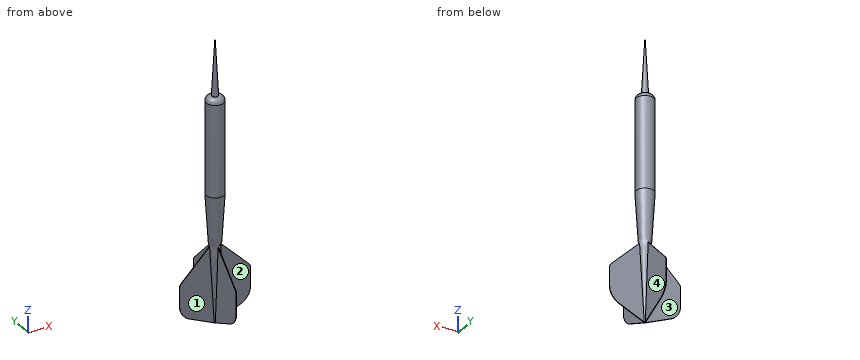
```python
from build123d import *

# Parameters (mm, degrees)
FLIGHT_DEPTH  = 0.125
FLIGHTS_COUNT = 4


with BuildPart() as part:
    # Sketch1 → Dart (revolve)
    with BuildSketch(Plane(origin=(0, 0, 0), x_dir=(0, 0, -1), z_dir=(1, 0, 0))):
        with BuildLine():
            Line((0, 0), (-32, 0))
            Line((-32, 0), (0, 1.75))
            ThreePointArc((0, 1.75), (0.787661698, 3.896312185), (2.887760572, 4.8))
            Line((2.887760572, 4.8), (52.94, 4.8))
            Line((52.94, 4.8), (122.94, 0.5))
            Line((122.94, 0.5), (122.94, 0))
            Line((122.94, 0), (0, 0))
        make_face()
    revolve(axis=Axis((0, 0, -122.94), (0, 0, 1)))

    # Sketch3 → Flight (add, symmetric)
    with BuildSketch(Plane(origin=(0, 0, 0), x_dir=(0, 0, -1), z_dir=(1, 0, 0))):
        with BuildLine():
            Line((77.94, 0), (96.561320344, 18.621320344))
            ThreePointArc((96.561320344, 18.621320344), (97.53459039, 19.271638598), (98.682640687, 19.5))
            Line((98.682640687, 19.5), (108.63598664, 19.5))
            ThreePointArc((108.63598664, 19.5), (113.537737955, 18.048035112), (116.857895759, 14.160629788))
            Line((116.857895759, 14.160629788), (122.94, 0.5))
            Line((122.94, 0.5), (122.94, 0))
            Line((122.94, 0), (77.94, 0))
        make_face()
    flight = extrude(amount=FLIGHT_DEPTH, both=True)

    # Flights: Flight ×4 about axis
    flights_axis = Axis((0, 0, 0), (0, 0, 1))
    for i in range(1, FLIGHTS_COUNT):
        add(flight.rotate(flights_axis, i * 360 / FLIGHTS_COUNT))


solid = part.part
```
Work out the finished part from the listing and answer in its coordinate system (mm). Face numbers are marked on the shaded views. A direction names the side the tool comes from. Give positions to 0.01 mm unless a question says otherwise; leave off trailing zeros. Write each loop counter-clockwise with the first axis right and the second up, starting at its lowest first coordinate (ties: lowest second). Pieces come first, ordered by that corner, then holes. Notation, with made-up numbers: (29.5, 51.5) - (86.5, 51.5) arc R27 cw to (86.5, 69.5) - close; hole circle Ø3 at (-27, -22). An arc over 180 degrees is marked (long way). Use one line per item in the form item = value.
1. Consider L1, parallel to Y at x = -8, z = -87 (3 decimals); L2, parallel to X at y = 0.5, z = -44. Determine where each line is inside the solid, lowest interval first.
Filled in:
L1 = -0.125 to 0.125
L2 = -4.77 to 4.77
2. A cutting plane is placed at A-A (y = 9.5). Write down the section's boundary in (x, z) (3 decimals).
Filled in:
outline = (-0.125, -118.933) - (0.125, -118.933) - (0.125, -87.44) - (-0.125, -87.44) - close
3. A cutting plane is placed at C-C (z = -38). Write down the section's boundary in (x, y).
Filled in:
outline = circle Ø9.6 at (0, 0)
4. For the marked faces 1, 2, 3 and 4, determine the directions among +Z, -Z, +X, -X, +Y, -Y from which every point of the face is accessible in a straight line to the end or side of a thin tool.
Filled in:
face_1 = -Z, -X, -Y
face_2 = -Z, +X, -Y
face_3 = -Z, -X, +Y
face_4 = -Z, +X, +Y
5. A cutting plane is placed at B-B (z = -75.5). Write down the section's boundary in (x, y), and give its area (3 significant figures).
Filled in:
outline = circle Ø6.83 at (0, 0)
area = 36.6 mm^2
6. A cutting plane is placed at D-D (y = 15.5). Write down the section's boundary in (x, z) (3 decimals), and give its area (3 significant figures).
Filled in:
outline = (-0.125, -116.119) - (0.125, -116.119) - (0.125, -93.44) - (-0.125, -93.44) - close
area = 5.67 mm^2
7. Each of these flat-tipped pins is pushed along its axis until it touches: pin 1 Ø9.5 at (x, z) = (-5.5, -111) entering from +Y; pin 2 Ø9.5 at (x, z) = (-12, -95) entering from -Y (3 decimals); pin 3 Ø5 at (x, z) = (-8, -82.5) entering from +Y (3 decimals); pin 4 Ø10 at (x, y) = (-14, -6.5) entering from +Z. Where does it stop, or does it pass through?
Filled in:
pin_1 = 1
pin_2 = -0.125
pin_3 = 0.125
pin_4 = through
